Design review of the part built by this model. Coordinates are the model's own, in mm. Coordinates: 2 decimals unless noted, no trailing zeros. Loops run counter-clockwise (first coordinate to the right, second up) from the corner with the lowest first, then second, coordinate; pieces in that order, holes last. Notation, with made-up numbers: M -2,-26.75 L 39,-26.75 A37 cw 39,9.25 Z; hole C 23.25,28 d10. An arc over 180 degrees is marked long. Write item = value, one per line. Start each with the question number.
```python
from build123d import *

# Parameters (mm, degrees)
PAD008_DEPTH    = 12.85
PAD009_DEPTH    = 10
SKETCH021_R     = 1.275
POCKET006_DEPTH = 15
SKETCH022_W     = 42
SKETCH022_H     = 4
POCKET007_DEPTH = 2
SKETCH027_R     = 1.3
POCKET011_DEPTH = 10
SKETCH028_W     = 10
SKETCH028_H     = 10
POCKET012_DEPTH = 22.8536497878


with BuildPart() as part:
    # Sketch012 (on DatumPlane) → Pad008 (new body)
    with BuildSketch(Plane(origin=(0.0007630761, 0.000154743, 17.0004579694), x_dir=(0.999999999, -4e-10, -4.48856e-05), z_dir=(-4.48856e-05, -9.1023e-06, -0.999999999))):
        with BuildLine():
            Line((0, 42), (42, 42))
            Line((42, 42), (42, -42))
            Line((42, -42), (0, -42))
            Line((0, -42), (0, -12.6))
            ThreePointArc((0, -12.6), (12.6, 0), (0, 12.6))
            Line((0, 42), (0, 12.6))
        make_face()
    extrude(amount=PAD008_DEPTH)

    # Sketch013 (on Face8 of Pad008) → Pad009 (join)
    with BuildSketch(Plane(origin=(0.0001862959, 3.77787e-05, 4.1504579829), x_dir=(0.999999999, -4e-10, -4.48856e-05), z_dir=(-4.48856e-05, -9.1023e-06, -0.999999999))):
        with BuildLine():
            ThreePointArc((0, -23.6), (23.6, 0), (0, 23.6))
            Line((0, 23.6), (0, 42))
            Line((0, 42), (42, 42))
            Line((42, 42), (42, -42))
            Line((42, -42), (0, -42))
            Line((0, -42), (0, -23.6))
        make_face()
    extrude(amount=PAD009_DEPTH)

    # Sketch021 (on Face7 of Pad009) → Pocket006 (cut)
    with BuildSketch(Plane(origin=(0.0007630761, 0.000154743, 17.0004579694), x_dir=(0, 1, -9.1023e-06), z_dir=(-0.999999999, 4e-10, 4.48856e-05))):
        with Locations((-37, 5)):
            Circle(SKETCH021_R)
        with Locations((37, 5)):
            Circle(SKETCH021_R)
    extrude(amount=-POCKET006_DEPTH, mode=Mode.SUBTRACT)

    # Sketch022 (on Face8 of Pocket006) → Pocket007 (cut)
    with BuildSketch(Plane(origin=(-0.0002625603, -5.32442e-05, -5.8495420067), x_dir=(0.999999999, -4e-10, -4.48856e-05), z_dir=(-4.48856e-05, -9.1023e-06, -0.999999999))):
        with Locations((21, 30)):
            Rectangle(SKETCH022_W, SKETCH022_H)
        with Locations((21, -30)):
            Rectangle(SKETCH022_W, SKETCH022_H)
    extrude(amount=-POCKET007_DEPTH, mode=Mode.SUBTRACT)

    # Sketch027 (on Face13 of Pocket007) → Pocket011 (cut)
    with BuildSketch(Plane(origin=(-0.0002625603, -5.32442e-05, -5.8495420067), x_dir=(0.999999999, -4e-10, -4.48856e-05), z_dir=(-4.48856e-05, -9.1023e-06, -0.999999999))):
        with Locations((32, 12.5)):
            Circle(SKETCH027_R)
        with Locations((32, -12.5)):
            Circle(SKETCH027_R)
    extrude(amount=-POCKET011_DEPTH, mode=Mode.SUBTRACT)

    # Sketch028 (on Face9 of Pocket011) → Pocket012 (cut, through all)
    with BuildSketch(Plane(origin=(-0.0002625603, -5.32442e-05, -5.8495420067), x_dir=(0.999999999, -4e-10, -4.48856e-05), z_dir=(-4.48856e-05, -9.1023e-06, -0.999999999))):
        with Locations((37, -37)):
            Rectangle(SKETCH028_W, SKETCH028_H)
        with Locations((37, 37)):
            Rectangle(SKETCH028_W, SKETCH028_H)
    extrude(amount=-POCKET012_DEPTH, mode=Mode.SUBTRACT)


solid = part.part
```
(1) Take a section at B-B (x = 39.5). State the section outline as (y, z) points.
(2) Take a section at A-A (y = 37). State the section outline as (x, z) points, plus the area to 3 significant figures.
(3) Take a section at C-C (z = 2.25). Give the number of separate pieces and of enclosed holes in the cut face, plus the area to 3 significant figures.
(4) Insertion check: pin 1 (5 mm diameter, centred on y = -35.5, z = 0, fed in from +X); pin 2 (1.6 mm diameter, centred on x = 32, y = 12.5, fed in from -Z). Each pin has a flat end and moves straight along its axis. Give the tip position at first contact, or say it passes through.
(5) Mouldability with a two-part tool opening along Z and no side actions: class faces 1 (the cylindrical face through (23.594, 0.519, -0.781)), 2 (the cylindrical face through (7.396, 35.726, 11.944)) as +Z half, -Z half, draft (parallel to the pull), parting line (faces both ways), or undercut.
(6) To check wall thickness, follow L1, parallel to Z at x = 37.5, y = 10; L2, parallel to Z at x = 12.5, y = 19; L3, parallel to Y at x = 10.5, z = 9.5. State the ranges of each line that lie inside material, in increasing order.
Results list:
q1.outline = M -32,-3.85 L -28,-3.85 L -28,-5.85 L 28,-5.85 L 28,-3.85 L 32,-3.85 L 32,17 L -32,17 Z
q2.outline = M 0,-5.85 L 32,-5.85 L 32,17 L 0,17 L 0,13.28 L 15,13.27 L 15,10.72 L 0,10.73 Z
q2.area = 693 mm^2
q3.separate_pieces = 1
q3.enclosed_holes = 2
q3.area = 2,440 mm^2
q4.pin_1 = 32
q4.pin_2 = 4.15
q5.face_1 = draft
q5.face_2 = undercut
q6.L1 = -5.85 to 17
q6.L2 = 4.15 to 17
q6.L3 = -42 to -6.97, 6.97 to 42
